from build123d import *

# Parameters (mm, degrees)
EXTRUDE_1_DEPTH     = 1500
CUT_EXTRUDE_4_DEPTH = 1500


with BuildPart() as part:
    # 草图2 → 凸台-拉伸1 (new body)
    with BuildSketch(Plane(origin=(0, 0, 0), x_dir=(1, 0, 0), z_dir=(0, 1, 0))):
        Polygon((345, 8.660254038), (180, 294.448637287), (165, 303.108891325), (-165, 303.108891325), (-180, 294.448637287), (-345, 8.660254038), (-345, -8.660254038), (-180, -294.448637287), (-165, -303.108891325), (165, -303.108891325), (180, -294.448637287), (345, -8.660254038), align=None)
    extrude(amount=EXTRUDE_1_DEPTH)

    # 草图5 → 切除-拉伸4 (cut)
    with BuildSketch(Plane(origin=(0, 0, 0), x_dir=(1, 0, 0), z_dir=(0, 1, 0))):
        with BuildLine():
            Line((238.21737139, 122.528375301), (345, 8.660254038))
            Line((345, 8.660254038), (379.520233023, 28.590519866))
            Line((379.520233023, 28.590519866), (334.34391274, 178.027059826))
            ThreePointArc((334.34391274, 178.027059826), (329.146090081, 190.032583711), (321.34791274, 200.536792121))
            Line((321.34791274, 200.536792121), (214.969297582, 314.638170659))
            Line((214.969297582, 314.638170659), (180, 294.448637287))
            Line((180, 294.448637287), (225.22137139, 145.038107596))
            ThreePointArc((225.22137139, 145.038107596), (230.419194049, 133.032583711), (238.21737139, 122.528375301))
        make_face()
        with BuildLine():
            Line((225.22137139, -145.038107596), (180, -294.448637287))
            Line((180, -294.448637287), (214.520233023, -314.378903115))
            Line((214.520233023, -314.378903115), (321.34791274, -200.536792121))
            ThreePointArc((321.34791274, -200.536792121), (329.146090081, -190.032583711), (334.34391274, -178.027059826))
            Line((334.34391274, -178.027059826), (379.969297582, -28.84978741))
            Line((379.969297582, -28.84978741), (345, -8.660254038))
            Line((345, -8.660254038), (238.21737139, -122.528375301))
            ThreePointArc((238.21737139, -122.528375301), (230.419194049, -133.032583711), (225.22137139, -145.038107596))
        make_face()
        with BuildLine():
            Line((12.996, 267.566482896), (165, 303.108891325))
            Line((165, 303.108891325), (165, 342.969422981))
            Line((165, 342.969422981), (12.996, 378.563851946))
            ThreePointArc((12.996, 378.563851946), (0, 380.065167421), (-12.996, 378.563851946))
            Line((-12.996, 378.563851946), (-165, 343.487958069))
            Line((-165, 343.487958069), (-165, 303.108891325))
            Line((-165, 303.108891325), (-12.996, 267.566482896))
            ThreePointArc((-12.996, 267.566482896), (0, 266.065167421), (12.996, 267.566482896))
        make_face()
        with BuildLine():
            Line((-12.996, -267.566482896), (-165, -303.108891325))
            Line((-165, -303.108891325), (-165, -342.969422981))
            Line((-165, -342.969422981), (-12.996, -378.563851946))
            ThreePointArc((-12.996, -378.563851946), (0, -380.065167421), (12.996, -378.563851946))
            Line((12.996, -378.563851946), (165, -343.487958069))
            Line((165, -343.487958069), (165, -303.108891325))
            Line((165, -303.108891325), (12.996, -267.566482896))
            ThreePointArc((12.996, -267.566482896), (0, -266.065167421), (-12.996, -267.566482896))
        make_face()
        with BuildLine():
            Line((-238.21737139, -122.528375301), (-345, -8.660254038))
            Line((-345, -8.660254038), (-379.520233023, -28.590519866))
            Line((-379.520233023, -28.590519866), (-334.34391274, -178.027059826))
            ThreePointArc((-334.34391274, -178.027059826), (-329.146090081, -190.032583711), (-321.34791274, -200.536792121))
            Line((-321.34791274, -200.536792121), (-214.969297582, -314.638170659))
            Line((-214.969297582, -314.638170659), (-180, -294.448637287))
            Line((-180, -294.448637287), (-225.22137139, -145.038107596))
            ThreePointArc((-225.22137139, -145.038107596), (-230.419194049, -133.032583711), (-238.21737139, -122.528375301))
        make_face()
        with BuildLine():
            Line((-225.22137139, 145.038107596), (-180, 294.448637287))
            Line((-180, 294.448637287), (-214.520233023, 314.378903115))
            Line((-214.520233023, 314.378903115), (-321.34791274, 200.536792121))
            ThreePointArc((-321.34791274, 200.536792121), (-329.14609008, 190.032583711), (-334.34391274, 178.027059826))
            Line((-334.34391274, 178.027059826), (-379.969297582, 28.84978741))
            Line((-379.969297582, 28.84978741), (-345, 8.660254038))
            Line((-345, 8.660254038), (-238.21737139, 122.528375301))
            ThreePointArc((-238.21737139, 122.528375301), (-230.419194049, 133.032583711), (-225.22137139, 145.038107596))
        make_face()
    extrude(amount=CUT_EXTRUDE_4_DEPTH, mode=Mode.SUBTRACT)


solid = part.part
CAD build for the part. Positions are in the model's coordinates, mm. A direction names the side the tool comes from. Round coordinates to 2 decimals unless told otherwise and drop trailing zeros. Write each loop counter-clockwise with the first axis right and the second up, starting at its lowest first coordinate (ties: lowest second). Pieces come first, ordered by that corner, then holes. Notation, with made-up numbers: M 4.25,-27 L 48.25,-27 A11 cw 48.25,-9 Z; hole C -10.75,4 d3. An arc over 180 degrees is marked long. Use a Markdown table: item, result. Add a question column.
1. Drill centre lines: probe 1 along X at (y, z) = (413, -91); probe 2 along Z at (x, y) = (-5, 772.5); probe 3 along X at (y, z) = (675.5, 96) (3 decimals). Where is each one in solid material? Low to high.
2. Slice it at C-C on x = 258.5. Give the cut face in (y, z), then the cut area to 3 significant figures.
3. Slice it at B-B on z = -79. Give the cut face in (x, y).
4. Pull direction X, two halves, no side cores. Call faces 1 (the face through (202.927, 739.5, 218.697)), 2 (the face through (90.062, 739.5, 285.586)), 3 (the face through (-90.062, 739.5, -285.586)), 4 (the face through (-292.356, 739.5, -64.797)): released by +X, released by -X, zero draft, split by the parting line, or undercut.
5. Slice it at A-A on y = 915. Give the cut face in (x, z).
6. 3-axis set-ups, long thin cutter, end or side, ignore diameter. For faces 5 (the face through (-87.93, 739.5, 285.09)), 6 (the face through (-5, 1500, -4)), 7 (the face through (87.93, 739.5, -285.09)): which of +Z, -Z, +X, -X, +Y, -Y reach the whole face in a straight line?
7. Flat gauge pins, fed straight in: P1, Ø12, axis at x = 90.5, y = 1225.5, coming from the -Z side; P2, Ø12, axis at y = 1319.5, z = 229.5, coming from the -X side; P3, Ø10, axis at y = 1221.5, z = 73.5, coming from the +X side. Where does each tip first touch, or does it go through?
Reply:
| question | item | result |
|---|---|---|
| 1 | probe 1 | x = -267.78 to 267.78 |
| 1 | probe 2 | z = -266.28 to 266.28 |
| 1 | probe 3 | x = -263.095 to 263.095 |
| 2 | outline | M 0,-100.9 L 1500,-100.9 L 1500,100.9 L 0,100.9 Z |
| 2 | area | 303,000 mm^2 |
| 3 | outline | M -279.04,0 L 279.04,0 L 279.04,1500 L -279.04,1500 Z |
| 4 | face 1 | released by +X |
| 4 | face 2 | undercut |
| 4 | face 3 | undercut |
| 4 | face 4 | released by -X |
| 5 | outline | M -345,-8.66 L -238.22,-122.53 A57 cw -225.22,-145.04 L -180,-294.45 L -165,-303.11 L -13,-267.57 A57 cw 13,-267.57 L 165,-303.11 L 180,-294.45 L 225.22,-145.04 A57 cw 238.22,-122.53 L 345,-8.66 L 345,8.66 L 238.22,122.53 A57 cw 225.22,145.04 L 180,294.45 L 165,303.11 L 13,267.57 A57 cw -13,267.57 L -165,303.11 L -180,294.45 L -225.22,145.04 A57 cw -238.22,122.53 L -345,8.66 Z |
| 6 | face 5 | +Z, +Y, -Y |
| 6 | face 6 | +Z, -Z, +X, -X, +Y |
| 6 | face 7 | -Z, +Y, -Y |
| 7 | P1 | stops at z = -287.09 |
| 7 | P2 | stops at x = -201.47 |
| 7 | P3 | stops at x = 288.88 |
